Design review of the part built by this model. Coordinates are the model's own, in mm. Coordinates: 2 decimals unless noted, no trailing zeros. Loops run counter-clockwise (first coordinate to the right, second up) from the corner with the lowest first, then second, coordinate; pieces in that order, holes last. Notation, with made-up numbers: (-16, -3) - (-12, -3) arc R11 cw to (-12, 18) - close; hole circle Ø4 at (57.5, 5). An arc over 180 degrees is marked (long way). Return JSON: item names as keys, results as strings. Group by question number.
from build123d import *

# Parameters (mm, degrees)
SKETCH_1_W           = 20
SKETCH_1_H           = 40
SKETCH_1_W_2         = 18
SKETCH_1_H_2         = 38
EXTRUDE_1_DEPTH      = 321
SKETCH_2_R           = 2.05
CUT_EXTRUDE_1_DEPTH  = 41
CUT_EXTRUDE_5_REACH  = 42
SKETCH_6_R           = 1.6
CUT_EXTRUDE_9_REACH  = 42
SKETCH_12_R          = 2.6
SKETCH_14_R          = 2.05
CUT_EXTRUDE_11_DEPTH = 41
SKETCH_15_R          = 2.525
CUT_EXTRUDE_12_DEPTH = 21
SKETCH_17_R          = 1.6
CUT_EXTRUDE_13_DEPTH = 21
SKETCH_18_R          = 9
CUT_EXTRUDE_14_DEPTH = 21


with BuildPart() as part:
    # 草图1 → 凸台-拉伸1 (new body)
    with BuildSketch(Plane(origin=(0, 0, 0), x_dir=(0, 0, -1), z_dir=(1, 0, 0))):
        Rectangle(SKETCH_1_W, SKETCH_1_H)
        Rectangle(SKETCH_1_W_2, SKETCH_1_H_2, mode=Mode.SUBTRACT)
    extrude(amount=EXTRUDE_1_DEPTH)

    # 草图2 → 切除-拉伸1 (cut, through all)
    with BuildSketch(Plane(origin=(0, 20, 0), x_dir=(1, 0, 0), z_dir=(0, 1, 0))):
        with Locations((76.5, 5)):
            Circle(SKETCH_2_R)
        with Locations((76.5, -5)):
            Circle(SKETCH_2_R)
        with Locations((104.5, -5)):
            Circle(SKETCH_2_R)
        with Locations((104.5, 5)):
            Circle(SKETCH_2_R)
        with Locations((216.5, -5)):
            Circle(SKETCH_2_R)
        with Locations((216.5, 5)):
            Circle(SKETCH_2_R)
        with Locations((244.5, -5)):
            Circle(SKETCH_2_R)
        with Locations((244.5, 5)):
            Circle(SKETCH_2_R)
    extrude(amount=-CUT_EXTRUDE_1_DEPTH, mode=Mode.SUBTRACT)

    # 草图6 → 切除-拉伸5 (cut, up to next)
    with BuildSketch(Plane.XZ.offset(20), mode=Mode.PRIVATE) as cut_extrude_5_sk1:
        with Locations((140.5, 6)):
            Circle(SKETCH_6_R)
    cut_extrude_5_tool1 = extrude(cut_extrude_5_sk1.sketch, amount=-CUT_EXTRUDE_5_REACH, mode=Mode.PRIVATE) & part.part
    add(cut_extrude_5_tool1.solids().sort_by_distance((140.5, -20, 6))[0], mode=Mode.SUBTRACT)
    # 草图6 → 切除-拉伸5 (cut, up to next)
    with BuildSketch(Plane.XZ.offset(20), mode=Mode.PRIVATE) as cut_extrude_5_sk2:
        with Locations((160.5, 6)):
            Circle(SKETCH_6_R)
    cut_extrude_5_tool2 = extrude(cut_extrude_5_sk2.sketch, amount=-CUT_EXTRUDE_5_REACH, mode=Mode.PRIVATE) & part.part
    add(cut_extrude_5_tool2.solids().sort_by_distance((160.5, -20, 6))[0], mode=Mode.SUBTRACT)
    # 草图6 → 切除-拉伸5 (cut, up to next)
    with BuildSketch(Plane.XZ.offset(20), mode=Mode.PRIVATE) as cut_extrude_5_sk3:
        with Locations((180.5, 6)):
            Circle(SKETCH_6_R)
    cut_extrude_5_tool3 = extrude(cut_extrude_5_sk3.sketch, amount=-CUT_EXTRUDE_5_REACH, mode=Mode.PRIVATE) & part.part
    add(cut_extrude_5_tool3.solids().sort_by_distance((180.5, -20, 6))[0], mode=Mode.SUBTRACT)
    # 草图6 → 切除-拉伸5 (cut, up to next)
    with BuildSketch(Plane.XZ.offset(20), mode=Mode.PRIVATE) as cut_extrude_5_sk4:
        with Locations((180.5, -6)):
            Circle(SKETCH_6_R)
    cut_extrude_5_tool4 = extrude(cut_extrude_5_sk4.sketch, amount=-CUT_EXTRUDE_5_REACH, mode=Mode.PRIVATE) & part.part
    add(cut_extrude_5_tool4.solids().sort_by_distance((180.5, -20, -6))[0], mode=Mode.SUBTRACT)
    # 草图6 → 切除-拉伸5 (cut, up to next)
    with BuildSketch(Plane.XZ.offset(20), mode=Mode.PRIVATE) as cut_extrude_5_sk5:
        with Locations((160.5, -6)):
            Circle(SKETCH_6_R)
    cut_extrude_5_tool5 = extrude(cut_extrude_5_sk5.sketch, amount=-CUT_EXTRUDE_5_REACH, mode=Mode.PRIVATE) & part.part
    add(cut_extrude_5_tool5.solids().sort_by_distance((160.5, -20, -6))[0], mode=Mode.SUBTRACT)
    # 草图6 → 切除-拉伸5 (cut, up to next)
    with BuildSketch(Plane.XZ.offset(20), mode=Mode.PRIVATE) as cut_extrude_5_sk6:
        with Locations((140.5, -6)):
            Circle(SKETCH_6_R)
    cut_extrude_5_tool6 = extrude(cut_extrude_5_sk6.sketch, amount=-CUT_EXTRUDE_5_REACH, mode=Mode.PRIVATE) & part.part
    add(cut_extrude_5_tool6.solids().sort_by_distance((140.5, -20, -6))[0], mode=Mode.SUBTRACT)

    # 草图12 → 切除-拉伸9 (cut, up to next)
    with BuildSketch(Plane(origin=(0, 20, 0), x_dir=(1, 0, 0), z_dir=(0, 1, 0)), mode=Mode.PRIVATE) as cut_extrude_9_sk1:
        with Locations((130.5, 0)):
            Circle(SKETCH_12_R)
    cut_extrude_9_tool1 = extrude(cut_extrude_9_sk1.sketch, amount=-CUT_EXTRUDE_9_REACH, mode=Mode.PRIVATE) & part.part
    add(cut_extrude_9_tool1.solids().sort_by_distance((130.5, 20, 0))[0], mode=Mode.SUBTRACT)
    # 草图12 → 切除-拉伸9 (cut, up to next)
    with BuildSketch(Plane(origin=(0, 20, 0), x_dir=(1, 0, 0), z_dir=(0, 1, 0)), mode=Mode.PRIVATE) as cut_extrude_9_sk2:
        with Locations((160.5, 0)):
            Circle(SKETCH_12_R)
    cut_extrude_9_tool2 = extrude(cut_extrude_9_sk2.sketch, amount=-CUT_EXTRUDE_9_REACH, mode=Mode.PRIVATE) & part.part
    add(cut_extrude_9_tool2.solids().sort_by_distance((160.5, 20, 0))[0], mode=Mode.SUBTRACT)
    # 草图12 → 切除-拉伸9 (cut, up to next)
    with BuildSketch(Plane(origin=(0, 20, 0), x_dir=(1, 0, 0), z_dir=(0, 1, 0)), mode=Mode.PRIVATE) as cut_extrude_9_sk3:
        with Locations((190.5, 0)):
            Circle(SKETCH_12_R)
    cut_extrude_9_tool3 = extrude(cut_extrude_9_sk3.sketch, amount=-CUT_EXTRUDE_9_REACH, mode=Mode.PRIVATE) & part.part
    add(cut_extrude_9_tool3.solids().sort_by_distance((190.5, 20, 0))[0], mode=Mode.SUBTRACT)

    # 草图14 → 切除-拉伸11 (cut, through all)
    with BuildSketch(Plane(origin=(0, 20, 0), x_dir=(1, 0, 0), z_dir=(0, 1, 0))):
        with Locations((314.5, 5)):
            Circle(SKETCH_14_R)
        with Locations((314.5, -5)):
            Circle(SKETCH_14_R)
        with Locations((286.5, -5)):
            Circle(SKETCH_14_R)
        with Locations((286.5, 5)):
            Circle(SKETCH_14_R)
        with Locations((34.5, -5)):
            Circle(SKETCH_14_R)
        with Locations((6.5, -5)):
            Circle(SKETCH_14_R)
        with Locations((6.5, 5)):
            Circle(SKETCH_14_R)
        with Locations((34.5, 5)):
            Circle(SKETCH_14_R)
    extrude(amount=-CUT_EXTRUDE_11_DEPTH, mode=Mode.SUBTRACT)

    # 草图15 → 切除-拉伸12 (cut, through all)
    with BuildSketch(Plane.XY.offset(10)):
        with Locations((145.5, 14)):
            Circle(SKETCH_15_R)
        with Locations((175.5, 14)):
            Circle(SKETCH_15_R)
    extrude(amount=-CUT_EXTRUDE_12_DEPTH, mode=Mode.SUBTRACT)

    # 草图17 → 切除-拉伸13 (cut, through all)
    with BuildSketch(Plane.XY.offset(10)):
        with Locations((12, 16.5)):
            Circle(SKETCH_17_R)
        with Locations((29, 16.5)):
            Circle(SKETCH_17_R)
        with Locations((12, -14)):
            Circle(SKETCH_17_R)
        with Locations((29, -14)):
            Circle(SKETCH_17_R)
        with Locations((43.5, -14)):
            Circle(SKETCH_17_R)
        with Locations((67.5, -14)):
            Circle(SKETCH_17_R)
        with Locations((222, -14)):
            Circle(SKETCH_17_R)
        with Locations((239, -14)):
            Circle(SKETCH_17_R)
        with Locations((253.5, -14)):
            Circle(SKETCH_17_R)
        with Locations((277.5, -14)):
            Circle(SKETCH_17_R)
        with Locations((292, -14)):
            Circle(SKETCH_17_R)
        with Locations((309, -14)):
            Circle(SKETCH_17_R)
        with Locations((82, -14)):
            Circle(SKETCH_17_R)
        with Locations((99, -14)):
            Circle(SKETCH_17_R)
        with Locations((292, 16.5)):
            Circle(SKETCH_17_R)
        with Locations((309, 16.5)):
            Circle(SKETCH_17_R)
        with Locations((150.5, -16)):
            Circle(SKETCH_17_R)
        with Locations((170.5, -16)):
            Circle(SKETCH_17_R)
    extrude(amount=-CUT_EXTRUDE_13_DEPTH, mode=Mode.SUBTRACT)

    # 草图18 → 切除-拉伸14 (cut, through all)
    with BuildSketch(Plane.XY.offset(10)):
        with Locations((138.5, -2)):
            Circle(SKETCH_18_R)
        with Locations((182.5, -2)):
            Circle(SKETCH_18_R)
    extrude(amount=-CUT_EXTRUDE_14_DEPTH, mode=Mode.SUBTRACT)


solid = part.part
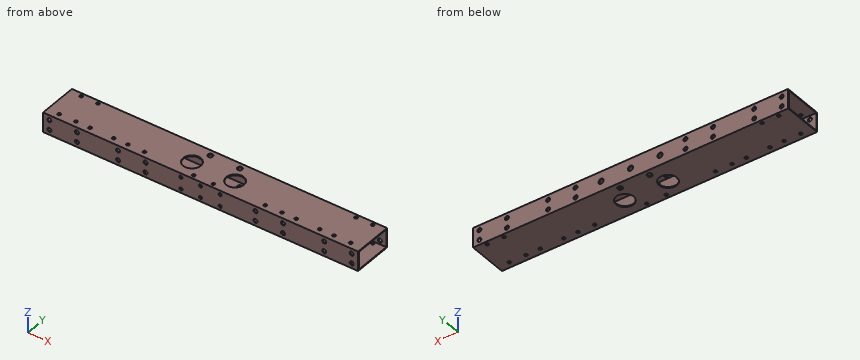
Item 1: Add section B-B (y = -6.5). State the section outline as (x, z) points.
Item 2: Add section A-A (x = 206.5). State the section outline as (y, z) points, then the cut area to 3 significant figures.
Item 3: To check wall thickness, follow line 1 (Z direction, x = 190.5, y = -18); line 2 (Y direction, x = 247, z = 8). State the ranges of each line that lie inside material, in increasing order. Write a range as from..to.
Item 4: For P1, Ø4, axis at x = 29, y = 16.5, coming from the +Z side, flat-tipped, find the tip position at first contact; note if it passes through.
Answers below:
{
 "1": {"outline": "(0, -10) - (130.71, -10) - (130.71, -9) - (0, -9) - close; (0, 9) - (130.71, 9) - (130.71, 10) - (0, 10) - close; (146.29, -10) - (174.71, -10) - (174.71, -9) - (146.29, -9) - close; (146.29, 9) - (174.71, 9) - (174.71, 10) - (146.29, 10) - close; (190.29, -10) - (321, -10) - (321, -9) - (190.29, -9) - close; (190.29, 9) - (321, 9) - (321, 10) - (190.29, 10) - close"},
 "2": {"outline": "(-20, -10) - (20, -10) - (20, 10) - (-20, 10) - close; hole (-19, -9) - (19, -9) - (19, 9) - (-19, 9) - close", "area": "116 mm^2"},
 "3": {"line 1": "z = -10..-9, 9..10", "line 2": "y = -20..-19, 19..20"},
 "4": {"P1": "stops at z = 10"}
}
